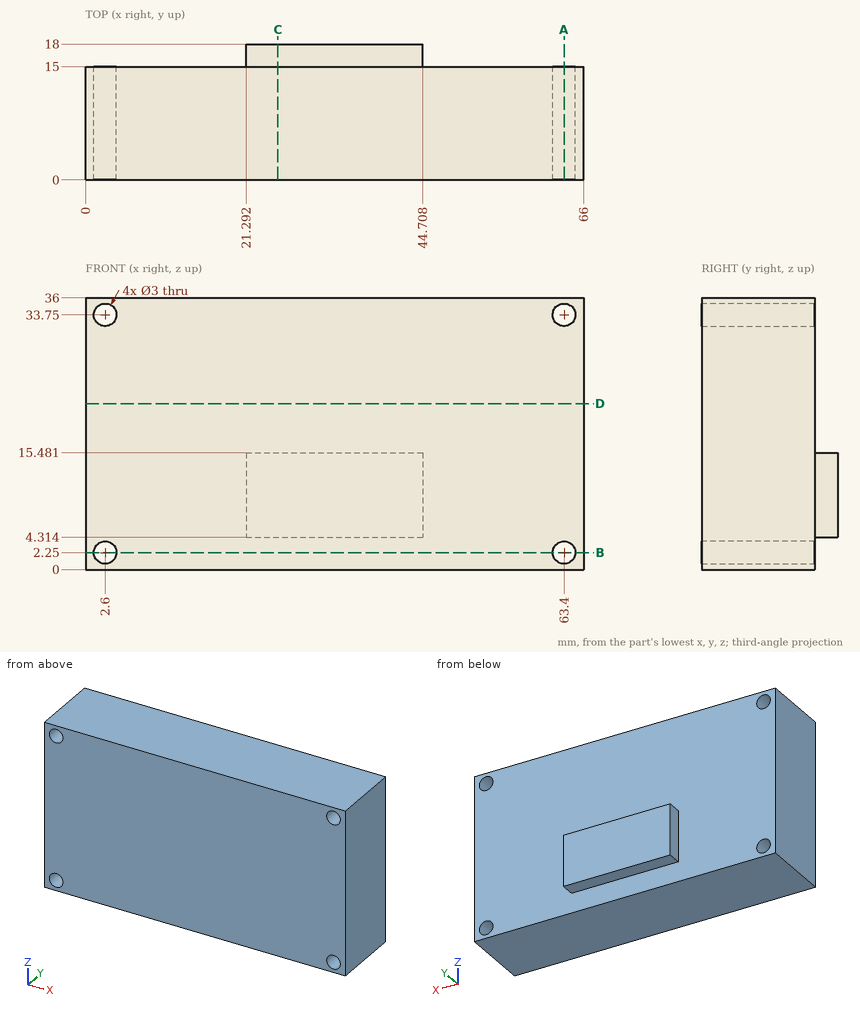
Job drawing, mm, ordinate dimensions from the low corner. One solid piece. Round coordinates to 2 decimals unless told otherwise and drop trailing zeros. Loops run counter-clockwise (first coordinate to the right, second up) from the corner with the lowest first, then second, coordinate; pieces in that order, holes last. Notation, with made-up numbers: (80.25, 32.25) -> (114.25, 32.25) arc R18 ccw to (114.25, 65.25) -> close; hole circle Ø11 at (55.25, 75.5). An arc over 180 degrees is marked (long way). Use a Markdown table: item, result.
1) Probe line 1 (X direction, y = 5, z = 33.75); line 2 (Z direction, x = 63.5, y = 5.25); line 3 (Y direction, x = 4, z = 3.5). List the from-to ranges inside material, lowest first. Write a range as [from, to].
The answers:
| item | result |
|---|---|
| line 1 | x = [0, 1.1], [4.1, 61.9], [64.9, 66] |
| line 2 | z = [0, 0.75], [3.75, 32.25], [35.25, 36] |
| line 3 | y = [0, 15] |
2) Drop flat-ended pins along their axis: pin 1 Ø1.5 at (y, z) = (16.5, 7.5) entering from -X; pin 2 Ø1.8 at (x, z) = (2.6, 33.75) entering from +Y; pin 3 Ø3.5 at (x, z) = (63.4, 33.75) entering from +Y; pin 4 Ø0.9 at (x, y) = (33.5, 16.5) entering from +Z. Give the stop position or say it passes through.
The answers:
| item | result |
|---|---|
| pin 1 | stops at x = 21.29 |
| pin 2 | passes through |
| pin 3 | stops at y = 15 |
| pin 4 | stops at z = 15.48 |
3) Cut at D-D, the plane z = 22. List the corners of the cut face in (x, y).
The answers:
| item | result |
|---|---|
| outline | (0, 0) -> (66, 0) -> (66, 15) -> (0, 15) -> close |
4) Cut at A-A, the plane x = 63.4. List the corners of the cut face in (y, z), and give its area (3 significant figures).
The answers:
| item | result |
|---|---|
| outline | (0, 0) -> (15, 0) -> (15, 0.75) -> (0, 0.75) -> close; (0, 3.75) -> (15, 3.75) -> (15, 32.25) -> (0, 32.25) -> close; (0, 35.25) -> (15, 35.25) -> (15, 36) -> (0, 36) -> close |
| area | 450 mm2 |
5) Cut at B-B, the plane z = 2.25. List the corners of the cut face in (x, y).
The answers:
| item | result |
|---|---|
| outline | (0, 0) -> (1.1, 0) -> (1.1, 15) -> (0, 15) -> close; (4.1, 0) -> (61.9, 0) -> (61.9, 15) -> (4.1, 15) -> close; (64.9, 0) -> (66, 0) -> (66, 15) -> (64.9, 15) -> close |
6) Cut at C-C, the plane x = 25.5. List the corners of the cut face in (y, z) (1 decimal).
The answers:
| item | result |
|---|---|
| outline | (0, 0) -> (15, 0) -> (15, 4.3) -> (18, 4.3) -> (18, 15.5) -> (15, 15.5) -> (15, 36) -> (0, 36) -> close |
